from build123d import *

# Parameters (mm, degrees)
SKETCH1_W               = 69.85
SKETCH1_H               = 31.75
BOSS_EXTRUDE1_DEPTH     = 24.88
CUT_EXTRUDE1_DEPTH      = 17.06
CUT_EXTRUDE2_DEPTH      = 7.82
CUT_EXTRUDE3_DEPTH      = 7.82
F_4_40_TAPPED_HOLE1_D   = 2.2606
SKETCH7_W               = 6.35
SKETCH7_H               = 31.75
BOSS_EXTRUDE2_DEPTH     = 1.778
SKETCH8_W               = 19.05
SKETCH8_H               = 18.53
CUT_EXTRUDE4_DEPTH      = 81.660395486
F_1_4_CLEARANCE_HOLE1_D = 7.14248


with BuildPart() as part:
    # Sketch1 → Boss-Extrude1 (new body)
    with BuildSketch(Plane.XY):
        with Locations((34.925, 15.875)):
            Rectangle(SKETCH1_W, SKETCH1_H)
    extrude(amount=BOSS_EXTRUDE1_DEPTH)

    # Sketch2 → Cut-Extrude1 (cut)
    with BuildSketch(Plane(origin=(0, 0, 0), x_dir=(-1, 0, 0), z_dir=(0, 0, -1))):
        with BuildLine():
            Line((-68.2625, 25.8953), (-50.8, 25.8953))
            Line((-50.8, 25.8953), (-50.8, 19.177))
            Line((-50.8, 19.177), (-25.4, 19.177))
            ThreePointArc((-25.4, 19.177), (-22.098, 15.875), (-25.4, 12.573))
            Line((-25.4, 12.573), (-50.8, 12.573))
            Line((-50.8, 12.573), (-50.8, 5.8547))
            Line((-50.8, 5.8547), (-68.2625, 5.8547))
            Line((-68.2625, 5.8547), (-68.2625, 25.8953))
        make_face()
    extrude(amount=-CUT_EXTRUDE1_DEPTH, mode=Mode.SUBTRACT)

    # Sketch3 → Cut-Extrude2 (cut)
    with BuildSketch(Plane.XY.offset(24.88)):
        with BuildLine():
            Line((29.068797257, 21.336), (40.781202743, 21.336))
            ThreePointArc((40.781202743, 21.336), (41.611202743, 20.992202743), (41.955, 20.162202743))
            Line((41.955, 20.162202743), (41.955, 11.587797257))
            ThreePointArc((41.955, 11.587797257), (41.611202743, 10.757797257), (40.781202743, 10.414))
            Line((40.781202743, 10.414), (29.068797257, 10.414))
            ThreePointArc((29.068797257, 10.414), (28.238797257, 10.757797257), (27.895, 11.587797257))
            Line((27.895, 11.587797257), (27.895, 20.162202743))
            ThreePointArc((27.895, 20.162202743), (28.238797257, 20.992202743), (29.068797257, 21.336))
        make_face()
    extrude(amount=-CUT_EXTRUDE2_DEPTH, mode=Mode.SUBTRACT)

    # Sketch4 → Cut-Extrude3 (cut)
    with BuildSketch(Plane.XY.offset(24.88)):
        Polygon((30.06348241, 31.75), (33.325, 23.876), (33.325, 21.336), (36.525, 21.336), (36.525, 23.876), (39.78651759, 31.75), align=None)
        Polygon((33.325, 10.414), (33.325, 7.874), (30.06348241, 0), (39.78651759, 0), (36.525, 7.874), (36.525, 10.414), align=None)
    extrude(amount=-CUT_EXTRUDE3_DEPTH, mode=Mode.SUBTRACT)

    # #4-40 Tapped Hole1 (through all)
    with Locations(Plane(origin=(0, 0, 17.06), x_dir=(-1, 0, 0), z_dir=(0, 0, -1))):
        with Locations((-44.45, 15.875), (-25.4, 15.875)):
            Hole(F_4_40_TAPPED_HOLE1_D / 2)

    # Sketch7 → Boss-Extrude2 (add)
    with BuildSketch(Plane(origin=(0, 0, 0), x_dir=(-1, 0, 0), z_dir=(0, 0, -1))):
        with Locations((-12.876533699, 15.875)):
            Rectangle(SKETCH7_W, SKETCH7_H)
    extrude(amount=BOSS_EXTRUDE2_DEPTH)

    # Sketch8 → Cut-Extrude4 (cut, through all)
    with BuildSketch(Plane(origin=(0, 31.75, 0), x_dir=(1, 0, 0), z_dir=(0, 1, 0))):
        with Locations((9.525, -15.615)):
            Rectangle(SKETCH8_W, SKETCH8_H)
    extrude(amount=-CUT_EXTRUDE4_DEPTH, mode=Mode.SUBTRACT)

    # 1/4 Clearance Hole1 (through all)
    with Locations(Plane.XY.offset(6.35)):
        with Locations((12.876533699, 15.875)):
            Hole(F_1_4_CLEARANCE_HOLE1_D / 2)


solid = part.part
The model under review builds one solid part; all positions refer to its coordinate system, in mm. A direction names the side the tool comes from. Coordinates: 2 decimals unless noted, no trailing zeros. Loops run counter-clockwise (first coordinate to the right, second up) from the corner with the lowest first, then second, coordinate; pieces in that order, holes last.
(1) Consider section B-B, the plane z = 22.5. Give the boundary of the cut face in (x, y) (3 decimals), plus the area to 3 significant figures.
Determined:
outline: (19.05, 0) - (30.063, 0) - (33.325, 7.874) - (33.325, 10.414) - (29.069, 10.414) arc R1.174 cw to (27.895, 11.588) - (27.895, 20.162) arc R1.174 cw to (29.069, 21.336) - (33.325, 21.336) - (33.325, 23.876) - (30.063, 31.75) - (19.05, 31.75) - close; (36.525, 7.874) - (39.787, 0) - (69.85, 0) - (69.85, 31.75) - (39.787, 31.75) - (36.525, 23.876) - (36.525, 21.336) - (40.781, 21.336) arc R1.174 cw to (41.955, 20.162) - (41.955, 11.588) arc R1.174 cw to (40.781, 10.414) - (36.525, 10.414) - close; hole circle Ø2.261 at (25.4, 15.875); hole circle Ø2.261 at (44.45, 15.875)
area: 1,330 mm2
(2) Insertion check: P1, Ø9.5, axis at x = 29.5, y = 15.5, coming from the -Z side; P2, Ø0.5, axis at y = 26.5, z = -0.5, coming from the +X side; P3, Ø1.4, axis at y = 24.5, z = -1, coming from the -X side. Each pin has a flat end and moves straight along its axis. Give the tip position at first contact, or say it passes through.
Determined:
P1: stops at z = 0
P2: stops at x = 16.05
P3: stops at x = 9.7
(3) Consider section D-D, the plane z = 4.5. Give the number of separate pieces and of enclosed holes in the cut face, plus the area to 3 significant figures.
Determined:
separate pieces: 1
enclosed holes: 2
area: 1,640 mm2
(4) Tool access review of faces 1 (the flat face through (50.8, 23, 8)), 2 (the flat face through (27.895, 16, 21)), 3 (the flat face through (9.702, 25, -1)): name each direction out of +Z, -Z, +X, -X, +Y, -Y from which nothing blocks a thin tool from reaching the whole face with its end or side.
Determined:
face 1: -Z
face 2: +Z
face 3: -Z, -X, +Y, -Y
(5) Consider section A-A, the plane x = 44.45. Give the boundary of the cut face in (y, z), plus the area to 3 significant figures.
Determined:
outline: (0, 0) - (12.57, 0) - (12.57, 17.06) - (14.74, 17.06) - (14.74, 24.88) - (0, 24.88) - close; (17.01, 17.06) - (19.18, 17.06) - (19.18, 0) - (31.75, 0) - (31.75, 24.88) - (17.01, 24.88) - close
area: 660 mm2
(6) Draft analysis for pull direction Y (two halves, no side actions). For faces 4 (the flat face through (33.325, 23, 21)), 5 (the flat face through (60, 25.895, 8)), 6 (the flat face through (38.133, 27.758, 21.025)), state which applies: +Y half, -Y half, draft (parallel to the pull), parting line (faces both ways), or undercut.
Determined:
face 4: draft
face 5: undercut
face 6: +Y half
(7) Wall thickness on L1, parallel to Y at x = 61, z = 8.75; L2, parallel to X at y = 6, z = 0.75; L3, parallel to Y at x = 44.45, z = 22.75: over which ranges is each line inside the solid? List them lowest first.
Determined:
L1: y = 0 to 5.85, 25.9 to 31.75
L2: x = 0 to 50.8, 68.26 to 69.85
L3: y = 0 to 14.74, 17.01 to 31.75
